Solid Edge part; units mm, degrees
sketch "Sketch1" plane through (0, 0, 0) normal (0, 0, 1) x (1, 0, 0)
  line L0 (-6.75, -7.25) -> (6.75, -7.25)
  line L1 (6.75, -7.25) -> (6.75, 7.25)
  line L2 (6.75, 7.25) -> (-6.75, 7.25)
  line L3 (-6.75, 7.25) -> (-6.75, -7.25)
  dimension "D1" = 6.75
  dimension "D2" = 6.75
extrude "Protrusion1" add sketch "Sketch1" along normal blind 1.6
sketch "Sketch2" plane through (0, 0, 1.6) normal (0, 0, 1) x (1, 0, 0)
  circle A0 centre (-5, -5.95) radius 0.5
  circle A1 centre (-2.5, -5.95) radius 0.5
  circle A2 centre (0, -5.95) radius 0.5
  circle A3 centre (2.5, -5.95) radius 0.5
  circle A4 centre (5, -5.95) radius 0.5
  dimension "D1" = 5
extrude "Cutout1" cut sketch "Sketch2" against normal through all
sketch "Sketch3" plane through (0, 0, 1.6) normal (0, 0, 1) x (1, 0, 0)
  line L0 (-6.75, 7.25) -> (6.75, 7.25)
  line L1 (6.75, 7.25) -> (6.75, -4.25)
  line L2 (6.75, -4.25) -> (-6.75, -4.25)
  line L3 (-6.75, -4.25) -> (-6.75, 7.25)
extrude "Extrusionsausprägung_2" add sketch "Sketch3" along normal blind 1.6
Here's how the part is built. I have some questions about the finished solid (model axes, mm). A direction names the side the tool comes from. Round coordinates to 2 decimals unless told otherwise and drop trailing zeros. Loops run counter-clockwise (first coordinate to the right, second up) from the corner with the lowest first, then second, coordinate; pieces in that order, holes last. Notation, with made-up numbers: (64.25, 36) -> (71.25, 36) arc R25 cw to (71.25, 72) -> close; hole circle Ø3 at (22, 73.5). An arc over 180 degrees is marked (long way). Answer as CSV lines item,"result". Start each with the question number.
1. Imagine slicing it at A-A on y = -5.95. Write out the boundary of the cut face in (x, z), plus the area to 3 significant figures.
2. Imagine slicing it at C-C on z = 0.7. Write out the boundary of the cut face in (x, y).
3. Imagine slicing it at B-B on x = 2.5. Write out the boundary of the cut face in (y, z).
4. If we mould it in two halves opening along X, with no side actions, what happens to faces 1 (the face through (0, 0, 0)), 2 (the face through (2.392, -6.438, 0.811)), 3 (the face through (6.75, 0, 2))? For each: pulls with the +X half, pulls with the -X half, needs draft (parallel to the pull), parting line crosses it, or undercut.
5. I'm going to push flat-ended pins straight in: P1, Ø1.5, axis at x = -3, z = 2.5, coming from the -Y side; P2, Ø2, axis at x = 3, y = -4, coming from the -Z side. Where does each tip first touch, or does it pass through?
6. Imagine slicing it at D-D on z = 2.7. Write out the boundary of the cut face in (x, y), plus the area to 3 significant figures.
7. For faces 4 (the face through (-0.108, -6.438, 0.811)), 5 (the face through (0, -4.25, 2)), which set-ups out of +Z, -Z, +X, -X, +Y, -Y let a thin tool reach every point of the face, with its end or its side?
8. I need wall thicknesses on probe 1 along Y at (x, z) = (5, 0.7); probe 2 along Y at (x, z) = (-3.75, 2.2); probe 3 along Z at (x, y) = (-4, -5.25). Which ranges of each line are inside material? Lowest first, please. Write a range as from..to.
Solution:
1,outline,"(-6.75, 0) -> (-5.5, 0) -> (-5.5, 1.6) -> (-6.75, 1.6) -> close; (-4.5, 0) -> (-3, 0) -> (-3, 1.6) -> (-4.5, 1.6) -> close; (-2, 0) -> (-0.5, 0) -> (-0.5, 1.6) -> (-2, 1.6) -> close; (0.5, 0) -> (2, 0) -> (2, 1.6) -> (0.5, 1.6) -> close; (3, 0) -> (4.5, 0) -> (4.5, 1.6) -> (3, 1.6) -> close; (5.5, 0) -> (6.75, 0) -> (6.75, 1.6) -> (5.5, 1.6) -> close"
1,area,"13.6 mm²"
2,outline,"(-6.75, -7.25) -> (6.75, -7.25) -> (6.75, 7.25) -> (-6.75, 7.25) -> close; hole circle Ø1 at (-5, -5.95); hole circle Ø1 at (-2.5, -5.95); hole circle Ø1 at (0, -5.95); hole circle Ø1 at (2.5, -5.95); hole circle Ø1 at (5, -5.95)"
3,outline,"(-7.25, 0) -> (-6.45, 0) -> (-6.45, 1.6) -> (-7.25, 1.6) -> close; (-5.45, 0) -> (7.25, 0) -> (7.25, 3.2) -> (-4.25, 3.2) -> (-4.25, 1.6) -> (-5.45, 1.6) -> close"
4,face 1,"needs draft"
4,face 2,"undercut"
4,face 3,"pulls with the +X half"
5,P1,"y = -4.25"
5,P2,"z = 0"
6,outline,"(-6.75, -4.25) -> (6.75, -4.25) -> (6.75, 7.25) -> (-6.75, 7.25) -> close"
6,area,"155 mm²"
7,face 4,"+Z, -Z"
7,face 5,"+Z, +X, -X, -Y"
8,probe 1,"-7.25..-6.45, -5.45..7.25"
8,probe 2,"-4.25..7.25"
8,probe 3,"0..1.6"
